from build123d import *

# Parameters (mm, degrees)
F1_DEPTH = 2.54
F2_DEPTH = 6.35


with BuildPart() as f1:
    # F0 (on Front) → F1 (new body)
    with BuildSketch(Plane.XZ):
        Polygon((14.4152494168, 36.1535907401), (5.6633852157, 1.778), (11.9867476806, 1.778), (16.2139723114, 15.2778414103), (21.2939723114, 15.2778414103), (26.0443502781, 1.778), (32.5503381746, 1.778), (23.4699654551, 36.1535907401), align=None)
        Polygon((21.2939723114, 20.6651952089), (16.2139723114, 20.6651952089), (18.7539723114, 27.8494001058), align=None, mode=Mode.SUBTRACT)
        Polygon((0, 0), (5.08, 0), (5.2107147535, 0), (5.6633852157, 1.778), (14.4152494168, 36.1535907401), (14.9956496651, 38.4332880643), (12.7460089281, 38.4314865499), (0, 38.4314865499), align=None)
        Polygon((32.5503381746, 1.778), (33.02, 0), (38.1, 0), (37.8601082237, 38.4515979446), (25.4348134573, 38.4416477567), (22.8661145367, 38.4395907401), (23.4699654551, 36.1535907401), align=None)
        Polygon((11.9867476806, 1.778), (11.43, 0), (26.67, 0), (26.0443502781, 1.778), (21.2939723114, 15.2778414103), (16.2139723114, 15.2778414103), align=None)
        Polygon((14.9956496651, 38.4332880643), (14.4152494168, 36.1535907401), (23.4699654551, 36.1535907401), (22.8661145367, 38.4395907401), align=None)
        Polygon((18.7539723114, 27.8494001058), (16.2139723114, 20.6651952089), (21.2939723114, 20.6651952089), align=None)
        Polygon((26.0443502781, 1.778), (26.67, 0), (33.02, 0), (32.5503381746, 1.778), align=None)
        Polygon((5.6633852157, 1.778), (5.2107147535, 0), (11.43, 0), (11.9867476806, 1.778), align=None)
    extrude(amount=-F1_DEPTH)

    # F0 (on Front) → F2 (join)
    with BuildSketch(Plane.XZ):
        Polygon((0, 0), (5.08, 0), (5.2107147535, 0), (5.6633852157, 1.778), (14.4152494168, 36.1535907401), (14.9956496651, 38.4332880643), (12.7460089281, 38.4314865499), (0, 38.4314865499), align=None)
        Polygon((18.7539723114, 27.8494001058), (16.2139723114, 20.6651952089), (21.2939723114, 20.6651952089), align=None)
        Polygon((32.5503381746, 1.778), (33.02, 0), (38.1, 0), (37.8601082237, 38.4515979446), (25.4348134573, 38.4416477567), (22.8661145367, 38.4395907401), (23.4699654551, 36.1535907401), align=None)
        Polygon((11.9867476806, 1.778), (11.43, 0), (26.67, 0), (26.0443502781, 1.778), (21.2939723114, 15.2778414103), (16.2139723114, 15.2778414103), align=None)
        Polygon((14.9956496651, 38.4332880643), (14.4152494168, 36.1535907401), (23.4699654551, 36.1535907401), (22.8661145367, 38.4395907401), align=None)
        Polygon((26.0443502781, 1.778), (26.67, 0), (33.02, 0), (32.5503381746, 1.778), align=None)
        Polygon((5.6633852157, 1.778), (5.2107147535, 0), (11.43, 0), (11.9867476806, 1.778), align=None)
    extrude(amount=F2_DEPTH)

    # F4 (on offset) → F5 (revolve)
    with BuildSketch(Plane.YZ.offset(19.05)):
        with BuildLine():
            ThreePointArc((-1.7915181816, 40.1749286294), (-2.9140501967, 37.4648966143), (-0.2040181816, 38.5874286294))
            ThreePointArc((-0.2040181816, 38.5874286294), (-0.6689861664, 39.7099606445), (-1.7915181816, 40.1749286294))
        make_face()
    revolve(axis=Axis((19.05, 1.9485244993, 41.7624286294), (0, 1, 0)))


solid = f1.part
Design review of the part built by this model. Coordinates are the model's own, in mm. A direction names the side the tool comes from. Coordinates: 2 decimals unless noted, no trailing zeros. Loops run counter-clockwise (first coordinate to the right, second up) from the corner with the lowest first, then second, coordinate; pieces in that order, holes last. Notation, with made-up numbers: M 50,45 L 54,45 A33 cw 54,84 Z; hole C 86.25,41.5 d2. An arc over 180 degrees is marked long. Answer as CSV lines item,"result".
Item 1: For probe 1 along X at (y, z) = (-2, 25.5); probe 2 along X at (y, z) = (-3.5, 23); probe 3 along X at (y, z) = (-4.25, 37.5), list the stretches that pass through material, from the lowest coordinate up.
Answer list:
probe 1,"0 to 11.7, 17.92 to 19.58, 26.28 to 37.94"
probe 2,"0 to 11.07, 17.04 to 20.47, 26.94 to 37.96"
probe 3,"0 to 37.87"
Item 2: Add section A-A on y = -5.25. State the section outline as (x, z) points.
Answer list:
outline,"M 0,0 L 38.1,0 L 37.86,38.45 L 12.75,38.43 L 0,38.43 Z; M 16.21,20.67 L 21.29,20.67 L 18.75,27.85 Z; hole M 5.66,1.78 L 11.99,1.78 L 16.21,15.28 L 21.29,15.28 L 26.04,1.78 L 32.55,1.78 L 23.47,36.15 L 14.42,36.15 Z"
Item 3: Add section D-D on x = 4.5. State the section outline as (y, z) points, plus the area to 3 significant figures.
Answer list:
outline,"M -6.35,0 L 2.54,0 L 2.54,38.43 L -6.35,38.43 Z"
area,"342 mm²"
Item 4: Add section C-C on z = 33.5. State the section outline as (x, y) points, plus the area to 3 significant figures.
Answer list:
outline,"M 0,-6.35 L 13.74,-6.35 L 13.74,0 L 24.17,0 L 24.17,-6.35 L 37.89,-6.35 L 37.89,2.54 L 0,2.54 Z"
area,"271 mm²"
Item 5: For P1, Ø1.5, axis at x = 18.5, y = 0, coming from the +Z side; P2, Ø5, axis at x = 28, y = -2.5, coming from the +Z side; P3, Ø1, axis at y = 0.5, z = 17.5, coming from the +X side, all flat-tipped, find the tip position at first contact; note any pin that passes through.
Answer list:
P1,"z = 46.11"
P2,"z = 38.45"
P3,"x = 37.99"
Item 6: Add section B-B on y = -0.75. State the section outline as (x, z) points, plus the area to 3 significant figures.
Answer list:
outline,"M 0,0 L 38.1,0 L 37.86,38.45 L 21.89,38.44 A4.37 ccw long 16.21,38.43 L 12.75,38.43 L 0,38.43 Z; M 16.21,20.67 L 21.29,20.67 L 18.75,27.85 Z; hole M 5.66,1.78 L 11.99,1.78 L 16.21,15.28 L 21.29,15.28 L 26.04,1.78 L 32.55,1.78 L 23.47,36.15 L 14.42,36.15 Z; hole C 19.05,41.76 d3.95"
area,"1,030 mm²"
Item 7: Machinability: for faces 5 (the face through (19, -6.35, 15)), 6 (the face through (28, -3, 19)), which of the approach directions +Z, -Z, +X, -X, +Y, -Y give a long, thin tool a straight path to every point of the face, cutting with its end or side? Answer none if there is none.
Answer list:
face 5,"+Z, -Z, +X, -X, -Y"
face 6,"-Y"
Item 8: The part is to be moulded in two halves that separate along X. For faces 1 (the face through (19, -2, 0)), 2 (the face through (20.04, -3.13, 24.21)), 3 (the face through (0, -2, 19)), 4 (the face through (19, -3, 15.278)), say which applies: pulls with the +X half, pulls with the -X half, needs draft (parallel to the pull), parting line crosses it, or undercut.
Answer list:
face 1,"needs draft"
face 2,"undercut"
face 3,"pulls with the -X half"
face 4,"undercut"
